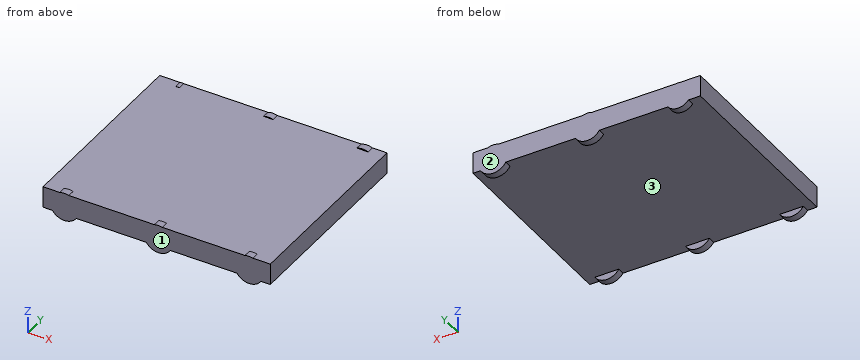
from build123d import *

# Parameters (mm, degrees)
F0_W     = 812.8
F0_H     = 76.2
F1_DEPTH = 698.5
F2_R     = 50.8
F3_DEPTH = 25.4
F5_R     = 52.824269
F5_R_2   = 51.150992
F5_R_3   = 47.107818
F6_DEPTH = 25.4


with BuildPart() as f1:
    # F0 (on Front) → F1 (new body)
    with BuildSketch(Plane.XZ):
        with Locations((131.72951, -4.131862)):
            Rectangle(F0_W, F0_H)
    extrude(amount=F1_DEPTH)

    # F2 (on face) → F3 (join)
    with BuildSketch(Plane.XZ.offset(698.5)):
        with Locations((461.92951, -14.740501)):
            Circle(F2_R)
        with Locations((137.779355, -14.777749)):
            Circle(F2_R)
        with Locations((-198.47049, -14.194834)):
            Circle(F2_R)
    extrude(amount=-F3_DEPTH)

    # F5 (on face) → F6 (join)
    with BuildSketch(Plane(origin=(0, 0, 0), x_dir=(-1, 0, 0), z_dir=(0, 1, 0))):
        with Locations((-465.801656, -14.819974)):
            Circle(F5_R)
        with Locations((-129.003808, -14.226768)):
            Circle(F5_R_2)
        with Locations((195.624262, -12.715756)):
            Circle(F5_R_3)
    extrude(amount=-F6_DEPTH)


solid = f1.part
Can you work these out from the model? Positions are in its coordinate system, mm. Face numbers are marked on the shaded views. Give positions to 0.01 mm unless a question says otherwise; leave off trailing zeros. Loops run counter-clockwise (first coordinate to the right, second up) from the corner with the lowest first, then second, coordinate; pieces in that order, holes last. Notation, with made-up numbers: M 86.5,-5 L 120.5,-5 A20 ccw 120.5,-1 Z; hole C -2.75,-23 d9. An arc over 180 degrees is marked long. One line per item, written item: value. Start each with the question number.
1) I'm going to push flat-ended pins straight in: pin 1 (10 mm diameter, centred on x = 222.5, y = -438.5, fed in from +Z); pin 2 (1.5 mm diameter, centred on x = -89, y = -121, fed in from -Z). Where does each tip first touch, or does it pass through?
2) If I drill on line 1 (Y direction, x = 135.5, z = -62.5); line 2 (Z direction, x = 292.5, y = -513), over which ranges is the centre line in solid material (lowest first)? Write a range as [from, to].
3) If we section it at B-B, the plane x = 70: Write out the boundary of the cut face in (y, z).
4) Thinking about a two-plate mould opening in Y: for the marked faces 1, 2 and 3, which applies, +Y half, -Y half, draft (parallel to the pull), parting line (faces both ways), or undercut?
5) If we section it at A-A, the plane y = -159.5: Write out the boundary of the cut face in (x, z).
Completed:
1. pin 1: stops at z = 33.97
1. pin 2: stops at z = -42.23
2. line 1: y = [-698.5, -673.1], [-25.4, 0]
2. line 2: z = [-42.23, 33.97]
3. outline: M -698.5,-42.23 L 0,-42.23 L 0,33.97 L -698.5,33.97 Z
4. face 1: -Y half
4. face 2: +Y half
4. face 3: undercut
5. outline: M -274.67,-42.23 L 538.13,-42.23 L 538.13,33.97 L -274.67,33.97 Z
